Source: CAD feature listing. Evaluate the final solid. Frame: model axes, mm. Coordinates: 2 decimals unless noted, no trailing zeros. Write each loop counter-clockwise with the first axis right and the second up, starting at its lowest first coordinate (ties: lowest second). Pieces come first, ordered by that corner, then holes. Notation, with made-up numbers: (49, 24.25) -> (89, 24.25) arc R19 ccw to (89, 58.25) -> close; hole circle Ø7 at (63, 43). An arc over 180 degrees is marked (long way). Write item = value, one per line.
from build123d import *

# Parameters (mm, degrees)
F0_W     = 155
F0_H     = 30
F1_DEPTH = 3
F2_D     = 3.3
F3_R     = 5
F4_R     = 1
F5_D     = 3.3


with BuildPart() as f1:
    # F0 (on Top) → F1 (new body)
    with BuildSketch(Plane.XY):
        Rectangle(F0_W, F0_H)
    extrude(amount=F1_DEPTH)

    # F2 (through all)
    with Locations(Plane(origin=(0, 0, 0), x_dir=(1, 0, 0), z_dir=(0, 0, -1))):
        with Locations((-67.5, 0), (67.5, 0)):
            Hole(F2_D / 2)

    # F3
    f3_edges = [f1.edges().sort_by_distance(p)[0] for p in [
        (-77.5, 15, 1.5),
        (-77.5, -15, 1.5),
        (77.5, -15, 1.5),
        (77.5, 15, 1.5),
    ]]
    fillet(f3_edges, radius=F3_R)

    # F4
    f4_edges = [f1.edges().sort_by_distance(p)[0] for p in [
        (0, -15, 3),
        (0, -15, 0),
    ]]
    fillet(f4_edges, radius=F4_R)

    # F5 (through all)
    with Locations(Plane(origin=(0, 0, 0), x_dir=(1, 0, 0), z_dir=(0, 0, -1))):
        with Locations((-33.3, 0), (33.3, 0)):
            Hole(F5_D / 2)


solid = f1.part
1) Cut plane B-B, the plane y = 0. Output: boundary loops of the cut face in (x, z).
Answer block:
outline = (-77.5, 1) arc R1 ccw to (-76.5, 0) -> (-69.15, 0) -> (-69.15, 3) -> (-76.5, 3) arc R1 ccw to (-77.5, 2) -> close; (-65.85, 0) -> (-34.95, 0) -> (-34.95, 3) -> (-65.85, 3) -> close; (-31.65, 0) -> (31.65, 0) -> (31.65, 3) -> (-31.65, 3) -> close; (34.95, 0) -> (65.85, 0) -> (65.85, 3) -> (34.95, 3) -> close; (69.15, 0) -> (76.5, 0) arc R1 ccw to (77.5, 1) -> (77.5, 2) arc R1 ccw to (76.5, 3) -> (69.15, 3) -> close
2) Cut plane A-A, the plane x = -67.5. Output: boundary loops of the cut face in (y, z), and give its area (3 significant figures).
Answer block:
outline = (-15, 1) arc R1 ccw to (-14, 0) -> (-1.65, 0) -> (-1.65, 3) -> (-14, 3) arc R1 ccw to (-15, 2) -> close; (1.65, 0) -> (14, 0) arc R1 ccw to (15, 1) -> (15, 2) arc R1 ccw to (14, 3) -> (1.65, 3) -> close
area = 79.2 mm2
3) Pull-direction query (X, two-part tool) for faces 1 (the cylindrical face through (-66.284, -1.115, 1.521)), 2 (the cylindrical face through (-76.07, -13.5, 1.51)), 3 (the cylindrical face through (76, -13.57, 1.51)), 4 (the cylindrical face through (34.95, -0.07, 1.52)); classes: +X half, -X half, draft (parallel to the pull), parting line (faces both ways), or undercut.
Answer block:
face_1 = undercut
face_2 = -X half
face_3 = +X half
face_4 = undercut
4) Material intervals for probe 1 along Y at (x, z) = (-67.5, 1.2); probe 2 along X at (y, z) = (-0.5, 0.7); probe 3 along Y at (x, z) = (66.5, 0.2), sorted ascending. Write a range as [from, to].
Answer block:
probe_1 = [-15, -1.65], [1.65, 15]
probe_2 = [-77.45, -69.07], [-65.93, -34.87], [-31.73, 31.73], [34.87, 65.93], [69.07, 77.45]
probe_3 = [-14.6, -1.31], [1.31, 14.6]
